Can you work these out from the model? Positions are in its coordinate system, mm. Give positions to 0.01 mm unless a question says otherwise; leave off trailing zeros. Loops run counter-clockwise (first coordinate to the right, second up) from the corner with the lowest first, then second, coordinate; pieces in that order, holes last.
from build123d import *

# Parameters (mm, degrees)
IZIM1_W                     = 104
IZIM1_H                     = 35
Y_KSEKLIK_EKSTR_ZYON1_DEPTH = 2
IZIM2_R                     = 1.5
KES_EKSTR_ZYON1_DEPTH       = 2
IZIM3_R                     = 2.5
KES_EKSTR_ZYON2_DEPTH       = 0.1
PAH2_SIZE                   = 1
IZIM4_R                     = 1.5
KES_EKSTR_ZYON3_DEPTH       = 2
IZIM5_R                     = 2.5
KES_EKSTR_ZYON4_DEPTH       = 0.1
PAH3_SIZE                   = 1
RADYUS1_R                   = 4
IZIM6_R                     = 4
IZIM6_W                     = 12
IZIM6_H                     = 8
KES_EKSTR_ZYON5_DEPTH       = 2
PAH4_SIZE                   = 1
PAH5_SIZE                   = 1


with BuildPart() as part:
    # Çizim1 → Yükseklik-Ekstrüzyon1 (new body)
    with BuildSketch(Plane.XY):
        with Locations((-52, 17.5)):
            Rectangle(IZIM1_W, IZIM1_H)
    extrude(amount=Y_KSEKLIK_EKSTR_ZYON1_DEPTH)

    # Çizim2 → Kes-Ekstrüzyon1 (cut)
    with BuildSketch(Plane.XY.offset(2)):
        with Locations((-100, 31)):
            Circle(IZIM2_R)
        with Locations((-100, 4)):
            Circle(IZIM2_R)
        with Locations(Location((-4, 4, 0), (0, 0, 180))):
            Circle(IZIM2_R)
        with Locations(Location((-4, 31, 0), (0, 0, 180))):
            Circle(IZIM2_R)
    extrude(amount=-KES_EKSTR_ZYON1_DEPTH, mode=Mode.SUBTRACT)

    # Çizim3 → Kes-Ekstrüzyon2 (cut)
    with BuildSketch(Plane.XY.offset(2)):
        with Locations((-100, 31)):
            Circle(IZIM3_R)
        with Locations((-100, 4)):
            Circle(IZIM3_R)
        with Locations(Location((-4, 4, 0), (0, 0, 180))):
            Circle(IZIM3_R)
        with Locations(Location((-4, 31, 0), (0, 0, 180))):
            Circle(IZIM3_R)
    extrude(amount=-KES_EKSTR_ZYON2_DEPTH, mode=Mode.SUBTRACT)

    # Pah2
    pah2_edges = [part.edges().sort_by_distance(p)[0] for p in [
        (-2.5, 31, 1.9),
        (-2.5, 4, 1.9),
        (-101.5, 4, 1.9),
        (-101.5, 31, 1.9),
    ]]
    chamfer(pah2_edges, length=PAH2_SIZE - 0.0001)  # a hair under: the kernel refuses the full size

    # Çizim4 → Kes-Ekstrüzyon3 (cut)
    with BuildSketch(Plane.XY.offset(2)):
        with Locations((-52, 31)):
            Circle(IZIM4_R)
        with Locations((-52, 4)):
            Circle(IZIM4_R)
    extrude(amount=-KES_EKSTR_ZYON3_DEPTH, mode=Mode.SUBTRACT)

    # Çizim5 → Kes-Ekstrüzyon4 (cut)
    with BuildSketch(Plane.XY.offset(2)):
        with Locations((-52, 31)):
            Circle(IZIM5_R)
        with Locations((-52, 4)):
            Circle(IZIM5_R)
    extrude(amount=-KES_EKSTR_ZYON4_DEPTH, mode=Mode.SUBTRACT)

    # Pah3
    pah3_edges = [part.edges().sort_by_distance(p)[0] for p in [
        (-53.5, 31, 1.9),
        (-53.5, 4, 1.9),
    ]]
    chamfer(pah3_edges, length=PAH3_SIZE - 0.0001)  # a hair under: the kernel refuses the full size

    # Radyus1
    radyus1_edges = [part.edges().sort_by_distance(p)[0] for p in [
        (0, 0, 1),
        (-104, 0, 1),
        (-104, 35, 1),
        (0, 35, 1),
    ]]
    fillet(radyus1_edges, radius=RADYUS1_R)

    # Çizim6 → Kes-Ekstrüzyon5 (cut)
    with BuildSketch(Plane.XY.offset(2)):
        with Locations((-82, 17.5)):
            Circle(IZIM6_R)
        with Locations((-52, 19)):
            Rectangle(IZIM6_W, IZIM6_H)
    extrude(amount=-KES_EKSTR_ZYON5_DEPTH, mode=Mode.SUBTRACT)

    # Pah4
    pah4_edges = [part.edges().sort_by_distance(p)[0] for p in [
        (-58, 19, 2),
        (-52, 15, 2),
        (-46, 19, 2),
        (-52, 23, 2),
    ]]
    chamfer(pah4_edges, length=PAH4_SIZE)

    # Pah5
    pah5_edges = [part.edges().sort_by_distance(p)[0] for p in [
        (-86, 17.5, 2),
    ]]
    chamfer(pah5_edges, length=PAH5_SIZE)


solid = part.part
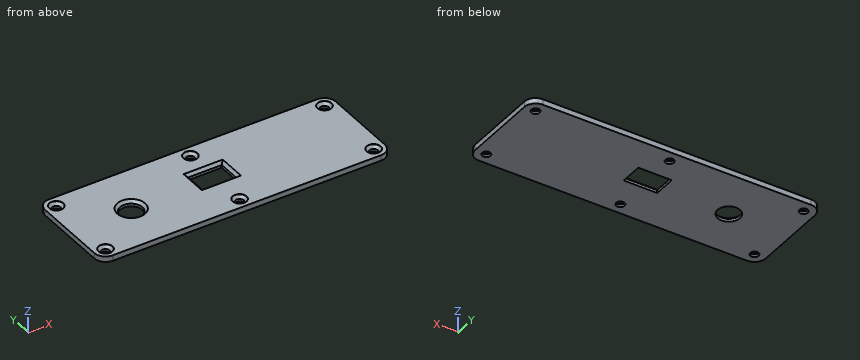
(1) Suppose I cut it at C-C on z = 0.5. Give the number of separate pieces and of enclosed holes in the cut face, plus the area to 3 significant figures.
Returned:
separate pieces: 1
enclosed holes: 8
area: 3,440 mm2
(2) Please list where these lines run through material, in increasing order: probe 1 along Y at (x, z) = (-52, 0.4); probe 2 along X at (y, z) = (3, 0.75); probe 3 along Y at (x, z) = (-52.5, 0.7).
Returned:
probe 1: y = 0 to 2.5, 5.5 to 15, 23 to 29.5, 32.5 to 35
probe 2: x = -103.87 to -101.12, -98.88 to -53.12, -50.88 to -5.12, -2.88 to -0.13
probe 3: y = 0 to 2.59, 5.41 to 15, 23 to 29.59, 32.41 to 35
(3) Suppose I cut it at A-A on x = -48. List the corners of the cut face in (y, z) for me, plus the area to 3 significant figures.
Returned:
outline: (0, 0) - (15, 0) - (15, 1) - (14, 2) - (0, 2) - close; (23, 0) - (35, 0) - (35, 2) - (24, 2) - (23, 1) - close
area: 53.0 mm2
(4) Suppose I cut it at B-B on y = 17.5. List the corners of the cut face in (x, z) for me, plus the area to 3 significant figures.
Returned:
outline: (-104, 0) - (-86, 0) - (-86, 1) - (-87, 2) - (-104, 2) - close; (-78, 0) - (-58, 0) - (-58, 1) - (-59, 2) - (-77, 2) - (-78, 1) - close; (-46, 0) - (0, 0) - (0, 2) - (-45, 2) - (-46, 1) - close
area: 166 mm2
(5) Will these pins go through, and if not, where does the flat tip stop? P1, Ø1.5, axis at x = -100.5, y = 32, coming from the +Z side; P2, Ø2.5, axis at x = -51, y = 4, coming from the +Z side; P3, Ø8, axis at x = -52, y = 31, coming from the +Z side; P4, Ø4, axis at x = -100, y = 4, coming from the +Z side.
Returned:
P1: stops at z = 1.27
P2: stops at z = 1.65
P3: stops at z = 2
P4: stops at z = 1.4
